Check sheet for the drawn part. Datum: minimum x, y, z corner. Units: mm. Coordinates: 2 decimals unless noted, no trailing zeros. Loops run counter-clockwise (first coordinate to the right, second up) from the corner with the lowest first, then second, coordinate; pieces in that order, holes last.
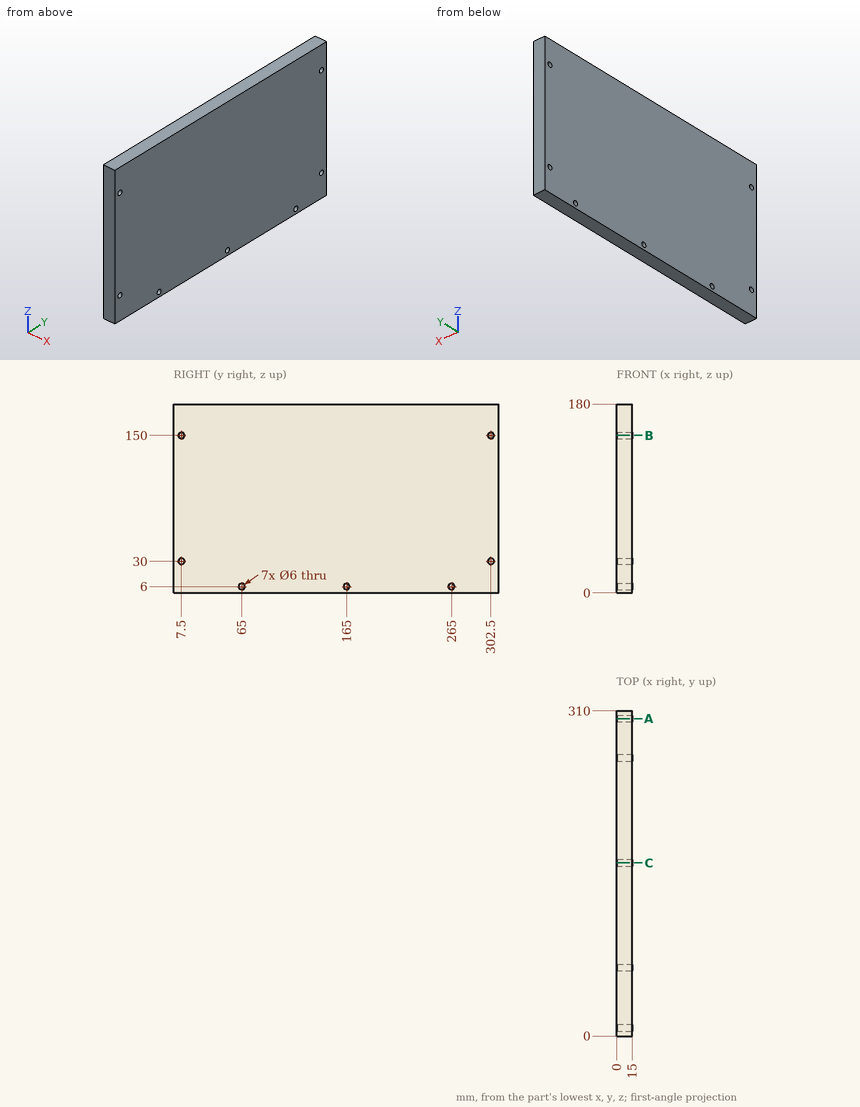
(1) Gauge pin test, flat end, axial feed: pin 1 Ø3.5 at (y, z) = (302.5, 30) entering from -X. Record the tip position at first contact, or that the pin passes through.
Findings:
pin 1: passes through
(2) Scan lines: L1, parallel to Z at x = 4.25, y = 7.5; L2, parallel to Y at x = 9, z = 150; L3, parallel to Z at x = 9.25, y = 65. Record each from-to range of solid material in increasing order.
Findings:
L1: z = 0 to 27, 33 to 147, 153 to 180
L2: y = 0 to 4.5, 10.5 to 299.5, 305.5 to 310
L3: z = 0 to 3, 9 to 180
(3) Sectioned sample at A-A on y = 302.5. Record the cut outline in (x, z), and give its area (3 significant figures).
Findings:
outline: (0, 0) - (15, 0) - (15, 27) - (0, 27) - close; (0, 33) - (15, 33) - (15, 147) - (0, 147) - close; (0, 153) - (15, 153) - (15, 180) - (0, 180) - close
area: 2,520 mm2
(4) Sectioned sample at B-B on z = 150. Record the cut outline in (x, y).
Findings:
outline: (0, 0) - (15, 0) - (15, 4.5) - (0, 4.5) - close; (0, 10.5) - (15, 10.5) - (15, 299.5) - (0, 299.5) - close; (0, 305.5) - (15, 305.5) - (15, 310) - (0, 310) - close
(5) Sectioned sample at C-C on y = 165. Record the cut outline in (x, z), and give its area (3 significant figures).
Findings:
outline: (0, 0) - (15, 0) - (15, 3) - (0, 3) - close; (0, 9) - (15, 9) - (15, 180) - (0, 180) - close
area: 2,610 mm2
